Model file for the job. Use its own axes, mm. A direction names the side the tool comes from. Round coordinates to 2 decimals unless told otherwise and drop trailing zeros. Order: outer loops, then holes, each group sorted by start corner. A loop starts at its lowest first (then second) coordinate and runs counter-clockwise, first axis right, second up. Notation, with made-up numbers: (23.25, 30) - (64.25, 30) arc R26 ccw to (64.25, 47) - close; hole circle Ø8 at (38.5, 55.25). An arc over 180 degrees is marked (long way). Answer as CSV lines item,"result". Start each with the question number.
1. Pull direction Z, two halves, no side cores. Call faces 5 (the face through (50.8, 22, 38)), 6 (the face through (63, 0, 38)), 7 (the face through (19, 13, 12.7)): released by +Z, released by -Z, zero draft, split by the parting line, or undercut.
2. Pin check, flat tips, straight feed: pin 1 Ø7 at (x, y) = (63.5, 23) entering from -Z; pin 2 Ø4 at (x, y) = (19.05, 12.7) entering from +Z; pin 3 Ø5.5 at (x, y) = (107.95, 12.7) entering from -Z; pin 4 Ø12.5 at (x, z) = (60.5, 34.5) entering from +Y. Stop position of each tip, or through.
3. Band-saw the part on B-B on x = 19.05. List the corners of the cut face in (y, z) (3 decimals).
4. 3-axis set-ups, long thin cutter, end or side, ignore diameter. For faces 1 (the face through (108, 13, 12.7)), 2 (the face through (0, 13, 38)), 3 (the face through (105.43, 10.77, 69.94)), 4 (the face through (63, 22, 50.8)): which of +Z, -Z, +X, -X, +Y, -Y reach the whole face in a straight line?
5. Band-saw the part on A-A on z = 34. List the corners of the cut face in (x, y).
6. Band-saw the part on C-C on y = 12.7. List the corners of the cut face in (x, z) (3 decimals), then the cut area to 3 significant figures.
7. Wall check: line 1 along Y through (x, z) = (19.05, 9.5) (3 decimals); line 2 along Z through (x, y) = (52, 21.25); line 3 along X through (y, z) = (24.5, 44). Give the ranges that are in metal, low to high. Write a range as [from, to].
```python
from build123d import *

# Parameters (mm, degrees)
SKETCH1_W           = 127
SKETCH1_H           = 25.4
BOSS_EXTRUDE1_DEPTH = 76.2
SKETCH2_R           = 3.175
CUT_EXTRUDE1_DEPTH  = 12.7
SKETCH3_R           = 3.175
CUT_EXTRUDE2_DEPTH  = 12.7
SKETCH4_W           = 25.4
SKETCH4_H           = 25.4
CUT_EXTRUDE3_DEPTH  = 6.35


with BuildPart() as part:
    # Sketch1 → Boss-Extrude1 (new body)
    with BuildSketch(Plane.XY):
        with Locations((63.5, 12.7)):
            Rectangle(SKETCH1_W, SKETCH1_H)
    extrude(amount=BOSS_EXTRUDE1_DEPTH)

    # Sketch2 → Cut-Extrude1 (cut)
    with BuildSketch(Plane.XY.offset(76.2)):
        with Locations((19.05, 12.7)):
            Circle(SKETCH2_R)
        with Locations((107.95, 12.7)):
            Circle(SKETCH2_R)
    extrude(amount=-CUT_EXTRUDE1_DEPTH, mode=Mode.SUBTRACT)

    # Sketch3 → Cut-Extrude2 (cut)
    with BuildSketch(Plane(origin=(0, 0, 0), x_dir=(-1, 0, 0), z_dir=(0, 0, -1))):
        with Locations((-107.95, 12.7)):
            Circle(SKETCH3_R)
        with Locations((-19.05, 12.7)):
            Circle(SKETCH3_R)
    extrude(amount=-CUT_EXTRUDE2_DEPTH, mode=Mode.SUBTRACT)

    # Sketch4 → Cut-Extrude3 (cut)
    with BuildSketch(Plane(origin=(0, 25.4, 0), x_dir=(1, 0, 0), z_dir=(0, 1, 0))):
        with Locations((63.5, -38.1)):
            Rectangle(SKETCH4_W, SKETCH4_H)
    extrude(amount=-CUT_EXTRUDE3_DEPTH, mode=Mode.SUBTRACT)


solid = part.part
```
Reply:
1,face 5,"undercut"
1,face 6,"zero draft"
1,face 7,"released by -Z"
2,pin 1,"stops at z = 0"
2,pin 2,"stops at z = 63.5"
2,pin 3,"stops at z = 12.7"
2,pin 4,"stops at y = 19.05"
3,outline,"(0, 0) - (9.525, 0) - (9.525, 12.7) - (15.875, 12.7) - (15.875, 0) - (25.4, 0) - (25.4, 76.2) - (15.875, 76.2) - (15.875, 63.5) - (9.525, 63.5) - (9.525, 76.2) - (0, 76.2) - close"
4,face 1,"-Z"
4,face 2,"+Z, -Z, -X, +Y, -Y"
4,face 3,"+Z"
4,face 4,"+Y"
5,outline,"(0, 0) - (127, 0) - (127, 25.4) - (76.2, 25.4) - (76.2, 19.05) - (50.8, 19.05) - (50.8, 25.4) - (0, 25.4) - close"
6,outline,"(0, 0) - (15.875, 0) - (15.875, 12.7) - (22.225, 12.7) - (22.225, 0) - (104.775, 0) - (104.775, 12.7) - (111.125, 12.7) - (111.125, 0) - (127, 0) - (127, 76.2) - (111.125, 76.2) - (111.125, 63.5) - (104.775, 63.5) - (104.775, 76.2) - (22.225, 76.2) - (22.225, 63.5) - (15.875, 63.5) - (15.875, 76.2) - (0, 76.2) - close"
6,area,"9,350 mm2"
7,line 1,"y = [0, 9.525], [15.875, 25.4]"
7,line 2,"z = [0, 25.4], [50.8, 76.2]"
7,line 3,"x = [0, 50.8], [76.2, 127]"
